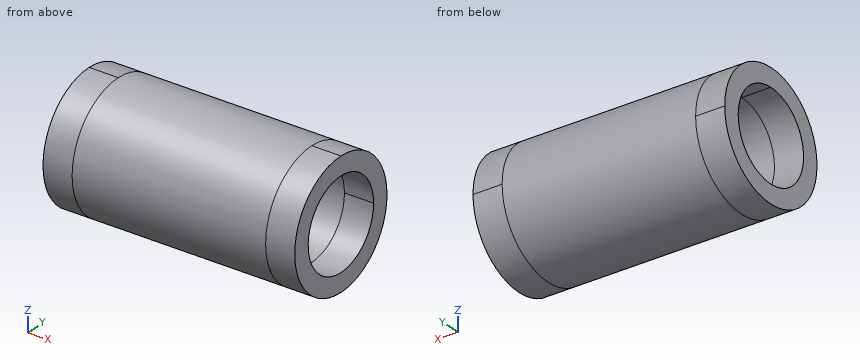
```python
from build123d import *

# Parameters (mm, degrees)
F1_W     = 17.6168819889
F1_H     = 11.0105499625
F5_R     = 37.8028899431
F5_R_2   = 26.7923399806
F6_DEPTH = 152.2524452932


# Not quite as in the source:
# - a pattern or mirror of a feature is missing from the dataset's text; its kind, count and spacing are read off the source's solid
# - the program builds the solid bodies; features that only make, move or delete a surface that nothing else refers to are left out


with BuildPart() as f2:
    # F1 (on Front) → F2 (revolve)
    with BuildSketch(Plane.XZ):
        with Locations((13.7020186521, 32.2976149619)):
            Rectangle(F1_W, F1_H)
    revolve(axis=Axis((44.2868806422, 0, 0), (1, 0, 0)))


with BuildPart() as f2_copies_1:
    # F2_copies: instance of F2
    add(f2.part.mirror(Plane(origin=(-53.615263, 0, 0), x_dir=(0, 0, -1), z_dir=(-1, 0, 0))))


with BuildPart() as f2_1:
    add(f2.part)

    add(f2_copies_1.part)  # F6 merges F2_copies_1
    # F5 (on face) → F6 (join, through all)
    with BuildSketch(Plane.YZ.offset(22.5104596466)):
        Circle(F5_R)
        Circle(F5_R_2, mode=Mode.SUBTRACT)
    extrude(amount=-F6_DEPTH)


solid = f2_1.part
```
CAD build for the part. Positions are in the model's coordinates, mm. Give positions to 0.01 mm unless a question says otherwise; leave off trailing zeros. Order: outer loops, then holes, each group sorted by start corner. A loop starts at its lowest first (then second) coordinate and runs counter-clockwise, first axis right, second up. Notation, with made-up numbers: M -19,84 L 27,84 A13 ccw 27,109 Z; hole C 2,88.5 d3. An arc over 180 degrees is marked long. Put each result on its own line as item: value. Start each with the question number.
(1) Drill centre lines: line 1 along Y through (x, z) = (-129.65, 0); line 2 along Z through (x, y) = (-114.5, 14). Where is each one in solid material? Low to high.
(2) Flat gauge pins, fed straight in: pin 1 Ø12 at (x, y) = (-21, -18.5) entering from -Z; pin 2 Ø4 at (x, y) = (-73.5, -5) entering from -Z; pin 3 Ø10 at (x, y) = (-58.5, -29.5) entering from +Z. Where does each tip first touch, or does it go through?
(3) Saw through at B-B, the plane x = -48. Write the cut outline in (y, z).
(4) Saw through at A-A, the plane z = -8. Write the cut outline in (x, y).
(5) Saw through at C-C, the plane y = 20.5. Write the cut outline in (x, z), then the cut area to 3 significant figures.
(6) Saw through at D-D, the plane z = -30. Write the cut outline in (x, y), then the cut area to 3 significant figures.
Check result:
1. line 1: y = -37.8 to -26.79, 26.79 to 37.8
1. line 2: z = -35.11 to -22.84, 22.84 to 35.11
2. pin 1: stops at z = -35.68
2. pin 2: stops at z = -37.68
2. pin 3: stops at z = 28.79
3. outline: C 0,0 d75.61; hole C 0,0 d53.58
4. outline: M -129.74,-36.95 L 22.51,-36.95 L 22.51,-25.57 L -129.74,-25.57 Z; M -129.74,25.57 L 22.51,25.57 L 22.51,36.95 L -129.74,36.95 Z
5. outline: M -129.74,-31.76 L 22.51,-31.76 L 22.51,-17.25 L -129.74,-17.25 Z; M -129.74,17.25 L 22.51,17.25 L 22.51,31.76 L -129.74,31.76 Z
5. area: 4,420 mm2
6. outline: M -129.74,-23 L 22.51,-23 L 22.51,23 L -129.74,23 Z
6. area: 7,000 mm2
